Work out the finished part from the listing and answer in its coordinate system (mm). Face numbers are marked on the shaded views. Coordinates: 2 decimals unless noted, no trailing zeros. Loops run counter-clockwise (first coordinate to the right, second up) from the corner with the lowest first, then second, coordinate; pieces in that order, holes last. Notation, with made-up numbers: (76, -23) -> (106, -23) arc R17 cw to (106, -12) -> close; hole circle Ø8 at (-39, 80). An arc over 180 degrees is marked (long way). Answer as CSV lines item,"result".
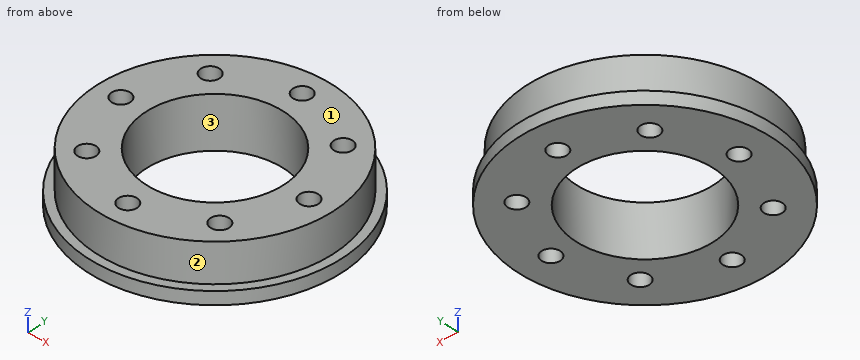
Autodesk Inventor part; units mm, degrees
ref_plane "YZ Plane" through (0, 0, 0) normal (1, 0, 0) x (0, 1, 0)
ref_plane "XZ Plane" through (0, 0, 0) normal (0, 1, 0) x (-1, 0, 0)
ref_plane "XY Plane" through (0, 0, 0) normal (0, 0, 1) x (1, 0, 0)
sketch "スケッチ1" plane through (0, 0, 0) normal (1, 0, 0) x (0, 1, 0)
  line L0 (16, 0) -> (27.5, 0)
  line L1 (27.5, 0) -> (27.5, -9)
  line L2 (27.5, -9) -> (29.5, -9)
  line L3 (29.5, -9) -> (29.5, -12)
  line L4 (16, -12) -> (16, 0)
  line L5 (0, -14.4) -> (0, 2.4)
  line L6 (29.5, -12) -> (16, -12)
  point P0 (0, 0)
  dimension "d5" = 9
  dimension "d30" = 2
  dimension "d31" = 27.5
  dimension "d32" = 3
  dimension "d33" = 16
revolve "回転1" add sketch "スケッチ1" angle 360 about axis through (0, 0, -10) along (0, 0, 1)
sketch "スケッチ2" plane through (0, 0, 0) normal (0, 0, 1) x (1, 0, 0)
  circle A0 centre (0, 0) radius 22
  point P0 (0, 22)
  point P1 (-15.5563, 15.5563)
  point P2 (-22, 0)
  point P3 (-15.5563, -15.5563)
  point P4 (0, -22)
  point P5 (15.5563, -15.5563)
  point P6 (22, 0)
  point P7 (15.5563, 15.5563)
  dimension "d11" = 44
  dimension "d14" = 360
hole "穴1" at (0, 22, 0) at (-15.5563, 15.5563, 0) at (-22, 0, 0) at (-15.5563, -15.5563, 0) at (0, -22, 0) at (15.5563, -15.5563, 0) at (22, 0, 0) at (15.5563, 15.5563, 0) direction (0, 0, -1) diameter 4.3 end through all
properties part number "base9"
(1) Consider line 1 along Y through (x, z) = (0, -4.25); line 2 along X through (y, z) = (-1, -8.5). Determine where each line is inside the solid, lowest interval first.
Computed values:
line 1,"-27.5 to -24.15, -19.85 to -16, 16 to 19.85, 24.15 to 27.5"
line 2,"-27.48 to -23.9, -20.1 to -15.97, 15.97 to 20.1, 23.9 to 27.48"
(2) For a pull along X with two mould halves and no side action, classify the marked faces 1, 2 and 3 as pulls with the +X half, pulls with the -X half, needs draft (parallel to the pull), parting line crosses it, or undercut.
Computed values:
face 1,"needs draft"
face 2,"parting line crosses it"
face 3,"undercut"
(3) A cutting plane is placed at C-C, the plane y = 10.5. Write down the section's boundary in (x, z).
Computed values:
outline,"(-27.57, -12) -> (-12.07, -12) -> (-12.07, 0) -> (-25.42, 0) -> (-25.42, -9) -> (-27.57, -9) -> close; (12.07, -12) -> (27.57, -12) -> (27.57, -9) -> (25.42, -9) -> (25.42, 0) -> (12.07, 0) -> close"
(4) Flat-ended cylindrical pins translate along their axes: pin 1 Ø4 at (x, y) = (-15.56, 15.56) entering from -Z; pin 2 Ø3 at (x, z) = (20, -1) entering from +Y; pin 3 Ø2 at (y, z) = (4.5, -10) entering from +X. Find the tip coordinate at first contact, or state that the pin passes through.
Computed values:
pin 1,"through"
pin 2,"y = 20.35"
pin 3,"x = 29.29"
(5) A cutting plane is placed at D-D, the plane x = -11. Write down the section's boundary in (y, z).
Computed values:
outline,"(-27.37, -12) -> (-11.62, -12) -> (-11.62, 0) -> (-25.2, 0) -> (-25.2, -9) -> (-27.37, -9) -> close; (11.62, -12) -> (27.37, -12) -> (27.37, -9) -> (25.2, -9) -> (25.2, 0) -> (11.62, 0) -> close"
(6) A cutting plane is placed at A-A, the plane x = 0. Write down the section's boundary in (y, z), and give its area (3 significant figures).
Computed values:
outline,"(-29.5, -12) -> (-24.15, -12) -> (-24.15, 0) -> (-27.5, 0) -> (-27.5, -9) -> (-29.5, -9) -> close; (-19.85, -12) -> (-16, -12) -> (-16, 0) -> (-19.85, 0) -> close; (16, -12) -> (19.85, -12) -> (19.85, 0) -> (16, 0) -> close; (24.15, -12) -> (29.5, -12) -> (29.5, -9) -> (27.5, -9) -> (27.5, 0) -> (24.15, 0) -> close"
area,"185 mm2"
